from build123d import *

# Parameters (mm, degrees)
SKETCH006_W     = 109
SKETCH006_H     = 65
SKETCH006_R     = 2.5
SKETCH006_R_2   = 6
SKETCH006_R_3   = 3.5
PAD_DEPTH       = 37.5
SKETCH010_W     = 21
SKETCH010_H     = 25.4
SKETCH010_W_2   = 15
POCKET_DEPTH    = 109
SKETCH011_W     = 41
SKETCH011_H     = 25.4
POCKET001_DEPTH = 29
SKETCH009_R     = 2.5
SKETCH009_R_2   = 6
POCKET002_DEPTH = 13
SKETCH008_R     = 4
POCKET003_DEPTH = 5
SKETCH001_R     = 5.4
POCKET004_DEPTH = 20
SKETCH007_R     = 13.05
POCKET005_DEPTH = 10


with BuildPart() as part:
    # Sketch006 → Pad (new body)
    with BuildSketch(Plane.YZ.offset(25)):
        with Locations((20.5, -10.5)):
            Rectangle(SKETCH006_W, SKETCH006_H)
        with Locations((-23.57, -36.07)):
            Circle(SKETCH006_R, mode=Mode.SUBTRACT)
        with Locations((23.57, -36.07)):
            Circle(SKETCH006_R, mode=Mode.SUBTRACT)
        with Locations((0, -12.5)):
            Circle(SKETCH006_R_2, mode=Mode.SUBTRACT)
        with Locations((25, -12.5)):
            Circle(SKETCH006_R_3, mode=Mode.SUBTRACT)
        with Locations((-25, -12.5)):
            Circle(SKETCH006_R_3, mode=Mode.SUBTRACT)
    extrude(amount=PAD_DEPTH)

    # Sketch010 → Pocket (cut)
    with BuildSketch(Plane(origin=(25, -34, 0), x_dir=(0, 0, -1), z_dir=(0, -1, 0))):
        with Locations((-11.5, 12.7)):
            Rectangle(SKETCH010_W, SKETCH010_H)
        with Locations((35.5, 12.7)):
            Rectangle(SKETCH010_W_2, SKETCH010_H)
    extrude(amount=-POCKET_DEPTH, mode=Mode.SUBTRACT)

    # Sketch011 → Pocket001 (cut)
    with BuildSketch(Plane(origin=(25, 0, -28), x_dir=(0, 1, 0), z_dir=(0, 0, -1))):
        with Locations((54.5, 12.7)):
            Rectangle(SKETCH011_W, SKETCH011_H)
    extrude(amount=-POCKET001_DEPTH, mode=Mode.SUBTRACT)

    # Sketch009 → Pocket002 (cut)
    with BuildSketch(Plane.YZ.offset(62.5)):
        with Locations((-23.57, 11.07)):
            Circle(SKETCH009_R)
        with Locations((23.57, 11.07)):
            Circle(SKETCH009_R)
        with Locations((62, -3)):
            Circle(SKETCH009_R_2)
    extrude(amount=-POCKET002_DEPTH, mode=Mode.SUBTRACT)

    # Sketch008 → Pocket003 (cut)
    with BuildSketch(Plane(origin=(50.4, 0, 0), x_dir=(0, 1, 0), z_dir=(-1, 0, 0))):
        with Locations((-23.57, -11.07)):
            Circle(SKETCH008_R)
        with Locations((23.57, -11.07)):
            Circle(SKETCH008_R)
        with Locations((-23.57, 36.07)):
            Circle(SKETCH008_R)
        with Locations((23.57, 36.07)):
            Circle(SKETCH008_R)
    extrude(amount=-POCKET003_DEPTH, mode=Mode.SUBTRACT)

    # Sketch001 → Pocket004 (cut)
    with BuildSketch(Plane.YZ.offset(62.5)):
        with Locations((-25, -12.5)):
            Circle(SKETCH001_R)
        with Locations((25, -12.5)):
            Circle(SKETCH001_R)
    extrude(amount=-POCKET004_DEPTH, mode=Mode.SUBTRACT)

    # Sketch007 → Pocket005 (cut)
    with BuildSketch(Plane.YZ.offset(62.5)):
        with Locations((0, -12.5)):
            Circle(SKETCH007_R)
    extrude(amount=-POCKET005_DEPTH, mode=Mode.SUBTRACT)


solid = part.part
The model under review builds one solid part; all positions refer to its coordinate system, in mm. A direction names the side the tool comes from. Round coordinates to 2 decimals unless told otherwise and drop trailing zeros. Loops run counter-clockwise (first coordinate to the right, second up) from the corner with the lowest first, then second, coordinate; pieces in that order, holes last. Notation, with made-up numbers: (35.25, 63) - (46.25, 63) arc R20 cw to (46.25, 81) - close; hole circle Ø11 at (-20.5, 85.5). An arc over 180 degrees is marked (long way). Use CSV: the item, a comma, the result in double quotes.
(1) Machinability: for faces 4 (the cylindrical face through (52.865, -24.091, -40.036)), 5 (the flat face through (52.5, 6, -15)), 6 (the cylindrical face through (33.628, -23.385, -15.605)), which of the approach directions +Z, -Z, +X, -X, +Y, -Y give a long, thin tool a straight path to every point of the face, cutting with its end or side? Answer none if there is none.
Working result:
face 4,"-X"
face 5,"+X"
face 6,"+X, -X"
(2) Take a section at B-B, the plane y = 0. Give the boundary of the cut face in (x, z).
Working result:
outline,"(25, -28) - (50.4, -28) - (50.4, -43) - (62.5, -43) - (62.5, -25.55) - (52.5, -25.55) - (52.5, -18.5) - (25, -18.5) - close; (25, -6.5) - (52.5, -6.5) - (52.5, 0.55) - (62.5, 0.55) - (62.5, 22) - (50.4, 22) - (50.4, 1) - (25, 1) - close"
(3) Take a section at D-D, the plane x = 60. State how many separate pieces and enclosed holes the cut face has, plus the area to 3 significant figures.
Working result:
separate pieces,"1"
enclosed holes,"8"
area,"6,180 mm^2"
(4) Take a section at C-C, the plane x = 48. Give the boundary of the cut face in (y, z), plus the area to 3 significant figures.
Working result:
outline,"(-34, -28) - (34, -28) - (34, 1) - (-34, 1) - close; hole circle Ø10.8 at (-25, -12.5); hole circle Ø12 at (0, -12.5); hole circle Ø10.8 at (25, -12.5)"
area,"1,680 mm^2"
(5) Clearance check with flat-ended pins moving along their axes: P1, Ø12, axis at x = 39, y = 27, coming from the +Z side; P2, Ø6, axis at y = 23.57, z = -36.07, coming from the -X side; P3, Ø6, axis at y = 17, z = 11, coming from the -X side. State where each tip first meets the part, or that it passes through.
Working result:
P1,"stops at z = 1"
P2,"stops at x = 55.4"
P3,"stops at x = 50.4"
(6) Take a section at A-A, the plane z = -36.07. Give the boundary of the cut face in (x, y), plus the area to 3 significant figures.
Working result:
outline,"(50.4, -34) - (62.5, -34) - (62.5, -26.07) - (55.4, -26.07) - (55.4, -27.57) - (50.4, -27.57) - close; (50.4, -19.57) - (55.4, -19.57) - (55.4, -21.07) - (62.5, -21.07) - (62.5, 21.07) - (55.4, 21.07) - (55.4, 19.57) - (50.4, 19.57) - close; (50.4, 27.57) - (55.4, 27.57) - (55.4, 26.07) - (62.5, 26.07) - (62.5, 75) - (50.4, 75) - close"
area,"1,170 mm^2"
(7) For line 1 (Y direction, x = 53.8, z = 11.07); line 2 (Y direction, x = 58, z = 11); line 3 (Y direction, x = 35.5, z = -12.5), list the stretches that pass through material, from the lowest coordinate up.
Working result:
line 1,"y = -34 to -27.57, -19.57 to 19.57, 27.57 to 75"
line 2,"y = -34 to -26.07, -21.07 to 21.07, 26.07 to 75"
line 3,"y = -34 to -28.5, -21.5 to -6, 6 to 21.5, 28.5 to 34"
(8) The part is to be moulded in two halves that separate along Z. For faces 1 (the flat face through (56, 75, -11)), 2 (the flat face through (38, 0, -28)), 3 (the cylindrical face through (52.64, -22.51, -17.29)), say which applies: pulls with the +Z half, pulls with the -Z half, needs draft (parallel to the pull), parting line crosses it, or undercut.
Working result:
face 1,"needs draft"
face 2,"pulls with the -Z half"
face 3,"undercut"
